Input: part model. Units: mm. Frame: model coordinates. A direction names the side the tool comes from. Round coordinates to 2 decimals unless told otherwise and drop trailing zeros. Order: outer loops, then holes, each group sorted by start corner. A loop starts at its lowest first (then second) coordinate and runs counter-clockwise, first axis right, second up. Notation, with made-up numbers: (57, 83.25) -> (90, 83.25) arc R21 ccw to (90, 95.25) -> close; hole circle Ø2 at (76.5, 68.5). An arc over 180 degrees is marked (long way). Use a Markdown table: item, result.
from build123d import *

# Parameters (mm, degrees)
F1_DEPTH = 45.212
F2_R     = 12.7
F3_DEPTH = 25.4
F4_SIZE  = 5.08


# Not quite as in the source:
# - a feature of the source that left no trace in its solid (it failed there, or was rolled back) is left out


with BuildPart() as f1:
    # F0 (on Right) → F1 (new body, symmetric)
    with BuildSketch(Plane.YZ):
        Polygon((24.4213882834, -39.0742197633), (24.4213882834, 44.8742993176), (0, 44.8742993176), (0, -19.2318409681), (-39.3794849515, -19.2318409681), (-39.3794849515, -39.0742197633), align=None)
    extrude(amount=F1_DEPTH, both=True)

    # F2 (on face) → F3 (cut)
    with BuildSketch(Plane(origin=(0, 24.4213882834, 0), x_dir=(-1, 0, 0), z_dir=(0, 1, 0))):
        with Locations((0, 6.7742993176)):
            Circle(F2_R)
    extrude(amount=-F3_DEPTH, mode=Mode.SUBTRACT)

    # F4
    f4_edges = [f1.edges().sort_by_distance(p)[0] for p in [
        (0, -39.379485, -19.231841),
    ]]
    chamfer(f4_edges, length=F4_SIZE)


solid = f1.part
1) Cut plane A-A on x = 0. Return loops of the section in (y, z), and give its area (3 significant figures).
Results found:
| item | result |
|---|---|
| outline | (-39.38, -39.07) -> (24.42, -39.07) -> (24.42, -5.93) -> (0, -5.93) -> (0, -19.23) -> (-34.3, -19.23) -> (-39.38, -24.31) -> close; (0, 19.47) -> (24.42, 19.47) -> (24.42, 44.87) -> (0, 44.87) -> close |
| area | 2,200 mm² |
2) Line query: L1, parallel to Z at x = 0, y = 5.25; L2, parallel to Y at x = 12, z = 36; L3, parallel to Z at x = -4.5, y = 20. Output: solid intervals per line, ascending. Write a range as [from, to].
Results found:
| item | result |
|---|---|
| L1 | z = [-39.07, -5.93], [19.47, 44.87] |
| L2 | y = [0, 24.42] |
| L3 | z = [-39.07, -5.1], [18.65, 44.87] |
3) Pin query (flat end, axial travel): pin 1 Ø10.5 at (x, y) = (-4.5, -13.5) entering from +Z; pin 2 Ø1.5 at (x, z) = (-9, 16) entering from -Y. Return the tip coordinate at first contact, or that it passes through.
Results found:
| item | result |
|---|---|
| pin 1 | stops at z = -19.23 |
| pin 2 | stops at y = 0 |
4) Pull-direction query (Z, two-part tool) for faces 1 (the flat face through (0.63, -36.88, -21.81)), 2 (the cylindrical face through (1.653, 12.382, 19.366)), 3 (the flat face through (1, -8, -39.074)), 4 (the flat face through (1, 24.421, -7)); classes: +Z half, -Z half, draft (parallel to the pull), parting line (faces both ways), or undercut.
Results found:
| item | result |
|---|---|
| face 1 | +Z half |
| face 2 | undercut |
| face 3 | -Z half |
| face 4 | draft |
5) Cut plane B-B on x = -39. Return loops of the section in (y, z), and give its area (3 significant figures).
Results found:
| item | result |
|---|---|
| outline | (-39.38, -39.07) -> (24.42, -39.07) -> (24.42, 44.87) -> (0, 44.87) -> (0, -19.23) -> (-34.3, -19.23) -> (-39.38, -24.31) -> close |
| area | 2,820 mm² |
6) Cut plane D-D on z = -11. Return loops of the section in (x, y).
Results found:
| item | result |
|---|---|
| outline | (-45.21, 0) -> (45.21, 0) -> (45.21, 24.42) -> (-45.21, 24.42) -> close |
7) Set-up query: faces 5 (the flat face through (1, -39.379, -32)), 6 (the flat face through (1, -17, -19.232)). Return all of +Z, -Z, +X, -X, +Y, -Y with unobstructed straight access to the full face (end or side cutting, diameter ignored); none if empty.
Results found:
| item | result |
|---|---|
| face 5 | +Z, -Z, +X, -X, -Y |
| face 6 | +Z, +X, -X, -Y |
8) Cut plane C-C on y = 19.5. Return loops of the section in (x, z).
Results found:
| item | result |
|---|---|
| outline | (-45.21, -39.07) -> (45.21, -39.07) -> (45.21, 44.87) -> (-45.21, 44.87) -> close; hole circle Ø25.4 at (0, 6.77) |
